from build123d import *

# Parameters (mm, degrees)
F0_W     = 101.6
F0_H     = 19.05
F2_DEPTH = 127
F1_W     = 63.5
F1_H     = 12.7
F3_DEPTH = 19.05
F4_R     = 5.08


with BuildPart() as f2:
    # F0 (on Front) → F2 (new body)
    with BuildSketch(Plane.XZ):
        Rectangle(F0_W, F0_H)
    extrude(amount=-F2_DEPTH)

    # F1 (on face) → F3 (cut)
    with BuildSketch(Plane.XZ):
        Rectangle(F1_W, F1_H)
    extrude(amount=-F3_DEPTH, mode=Mode.SUBTRACT)

    # F4
    f4_edges = [f2.edges().sort_by_distance(p)[0] for p in [
        (-50.8, 63.5, 9.525),
        (50.8, 63.5, 9.525),
        (50.8, 63.5, -9.525),
        (-50.8, 63.5, -9.525),
    ]]
    fillet(f4_edges, radius=F4_R)


solid = f2.part
Input: part model. Units: mm. Frame: model coordinates. A direction names the side the tool comes from. Give positions to 0.01 mm unless a question says otherwise; leave off trailing zeros. Order: outer loops, then holes, each group sorted by start corner. A loop starts at its lowest first (then second) coordinate and runs counter-clockwise, first axis right, second up. Notation, with made-up numbers: (-15, -5.5) - (-4, -5.5) arc R17 cw to (-4, 14.5) - close; hole circle Ø4 at (86.5, 28). An arc over 180 degrees is marked (long way). Write each question's results on one line, items separated by ' | '.
Item 1: Section B-B (x = 5.5). Return loops of the section in (y, z) (3 decimals).
A:
outline: (0, -9.525) - (127, -9.525) - (127, 9.525) - (0, 9.525) - (0, 6.35) - (19.05, 6.35) - (19.05, -6.35) - (0, -6.35) - close
Item 2: Draft query along X for faces 3 (the cylindrical face through (-49.35, 64.39, 8)), 4 (the cylindrical face through (49.27, 64.39, -8.08)), 5 (the flat face through (-0.7, 0, 6.5)), 6 (the flat face through (0, 9, -6.35)). Return one class per face: released by +X, released by -X, zero draft, split by the parting line, or undercut.
A:
face 3: released by -X | face 4: released by +X | face 5: zero draft | face 6: undercut
Item 3: Access query for faces 1 (the flat face through (-1, 63, 9.525)), 2 (the flat face through (0, 19.05, 0)). Directions: +Z, -Z, +X, -X, +Y, -Y. A direction counts if a zero-diameter tool reaches every point of the face in a straight line with its end or side. Return the directions, or none.
A:
face 1: +Z, +X, -X, +Y, -Y | face 2: -Y
Item 4: Section A-A (z = -1.5). Return loops of the section in (x, y), and give its area (3 significant figures).
A:
outline: (-50.8, 0) - (-31.75, 0) - (-31.75, 19.05) - (31.75, 19.05) - (31.75, 0) - (50.8, 0) - (50.8, 127) - (-50.8, 127) - close | area: 11,700 mm^2
Item 5: Material intervals for line 1 along Z through (x, y) = (-11, 6) (3 decimals); line 2 along X through (y, z) = (7, -4.5); line 3 along Y through (x, z) = (25, 1.5), sorted ascending.
A:
line 1: z = -9.525 to -6.35, 6.35 to 9.525 | line 2: x = -50.8 to -31.75, 31.75 to 50.8 | line 3: y = 19.05 to 127
Item 6: Contact query for flat-ended pins moving along their axis: pin 1 Ø1.5 at (y, z) = (87.5, 7.5) entering from -X; pin 2 Ø6.5 at (x, z) = (7, 0) entering from -Y. Output: stop coordinate, or through.
A:
pin 1: stops at x = -50.25 | pin 2: stops at y = 19.05
